Read the model definition and answer for the solid it produces. Units are mm, in the model's axes. Face numbers are marked on the shaded views. A direction names the side the tool comes from. Coordinates: 2 decimals unless noted, no trailing zeros. Loops run counter-clockwise (first coordinate to the right, second up) from the corner with the lowest first, then second, coordinate; pieces in that order, holes last. Notation, with made-up numbers: (51, -16) - (56, -16) arc R7 cw to (56, -10) - close; hole circle Ø11 at (76.5, -23). An arc over 180 degrees is marked (long way). Use one line per item in the form item = value.
from build123d import *

# Parameters (mm, degrees)
SKETCH1_W           = 30.86
SKETCH1_H           = 42.11
BOSS_EXTRUDE1_DEPTH = 10
SHELL2_T            = -2
SKETCH4_W           = 19.06
SKETCH4_H           = 2
CUT_EXTRUDE1_DEPTH  = 4
FILLET1_R           = 0.25
SKETCH5_R           = 1.5
CUT_EXTRUDE2_DEPTH  = 28.953495756
SKETCH6_R           = 1.5
CUT_EXTRUDE3_DEPTH  = 28.953495756


with BuildPart() as part:
    # Sketch1 → Boss-Extrude1 (new body)
    with BuildSketch(Plane(origin=(0, 0, 0), x_dir=(1, 0, 0), z_dir=(0, 1, 0))):
        Rectangle(SKETCH1_W, SKETCH1_H)
    extrude(amount=BOSS_EXTRUDE1_DEPTH)

    # Shell2
    shell2_openings = [part.faces().sort_by_distance(p)[0] for p in [
        (0, 10, 0),
    ]]
    offset(amount=SHELL2_T, openings=shell2_openings, kind=Kind.INTERSECTION)

    # Sketch4 → Cut-Extrude1 (cut)
    with BuildSketch(Plane(origin=(0, 10, 0), x_dir=(1, 0, 0), z_dir=(0, 1, 0))):
        with Locations((-3.9, -20.055)):
            Rectangle(SKETCH4_W, SKETCH4_H)
    extrude(amount=-CUT_EXTRUDE1_DEPTH, mode=Mode.SUBTRACT)

    # Fillet1
    fillet1_edges = [part.edges().sort_by_distance(p)[0] for p in [
        (0, 0, 21.055),
        (-15.43, 0, 0),
        (0, 0, -21.055),
        (15.43, 0, 0),
        (15.43, 5, 21.055),
        (-15.43, 5, 21.055),
        (-15.43, 5, -21.055),
        (15.43, 5, -21.055),
    ]]
    fillet(fillet1_edges, radius=FILLET1_R)

    # Sketch5 → Cut-Extrude2 (cut, through all)
    with BuildSketch(Plane.XZ):
        with Locations(Location((3.955545026, 15.646822422, 0), (0, 0, 270))):
            Circle(SKETCH5_R)
    extrude(amount=-CUT_EXTRUDE2_DEPTH, mode=Mode.SUBTRACT)

    # Sketch6 → Cut-Extrude3 (cut, through all)
    with BuildSketch(Plane.XZ):
        with Locations(Location((8.578599531, 12.725824803, 0), (0, 0, 270))):
            Circle(SKETCH6_R)
    extrude(amount=-CUT_EXTRUDE3_DEPTH, mode=Mode.SUBTRACT)


solid = part.part
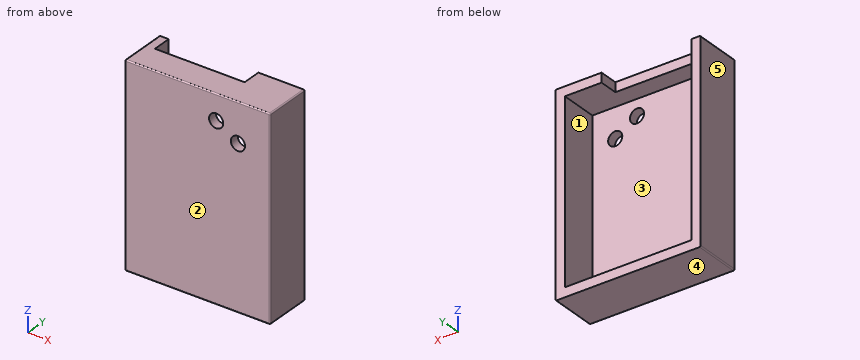
Item 1: Which of the six approach directions +Z, -Z, +X, -X, +Y, -Y give full straight-line access (tool end or side, diameter ignored) to the marked faces 1 and 2?
Results below:
face_1 = +Y
face_2 = +Z, -Z, +X, -X, -Y
Item 2: Each of these flat-tipped pins is pushed along its axis until it touches: P1, Ø5, axis at x = 8.58, z = 12.73, coming from the +Y side; P2, Ø1, axis at x = -7, z = 20, coming from the +Y side. Where does it stop, or does it pass through?
Results below:
P1 = 2
P2 = 6
Item 3: The part is cut by section B-B on y = 8.25. Give the vertices of the cut face in (x, z) (3 decimals).
Results below:
outline = (-15.43, -20.805) arc R0.25 ccw to (-15.18, -21.055) - (15.18, -21.055) arc R0.25 ccw to (15.43, -20.805) - (15.43, 20.805) arc R0.25 ccw to (15.18, 21.055) - (5.63, 21.055) - (5.63, 19.055) - (13.43, 19.055) - (13.43, -19.055) - (-13.43, -19.055) - (-13.43, 21.055) - (-15.18, 21.055) arc R0.25 ccw to (-15.43, 20.805) - close
Item 4: Find the intervals of material crossed by L1, parallel to X at y = 9.5, z = -18.5; L2, parallel to Z at x = 11, y = 7.25 (3 decimals); L3, parallel to Z at x = -1, y = 9.25 (3 decimals), in increasing order.
Results below:
L1 = -15.43 to -13.43, 13.43 to 15.43
L2 = -21.055 to -19.055, 19.055 to 21.055
L3 = -21.055 to -19.055
Item 5: For a pull along X with two mould halves and no side action, classify the marked faces 3, 4 and 5 as +X half, -X half, draft (parallel to the pull), parting line (faces both ways), or undercut.
Results below:
face_3 = undercut
face_4 = draft
face_5 = -X half
Item 6: The part is cut by section D-D on z = 7.5. Give the vertices of the cut face in (x, y), plus the area to 3 significant figures.
Results below:
outline = (-15.43, 0.25) arc R0.25 ccw to (-15.18, 0) - (15.18, 0) arc R0.25 ccw to (15.43, 0.25) - (15.43, 10) - (13.43, 10) - (13.43, 2) - (-13.43, 2) - (-13.43, 10) - (-15.43, 10) - close
area = 93.7 mm²
Item 7: The part is cut by section A-A on y = 3.75. Give the vertices of the cut face in (x, z) (3 decimals).
Results below:
outline = (-15.43, -20.805) arc R0.25 ccw to (-15.18, -21.055) - (15.18, -21.055) arc R0.25 ccw to (15.43, -20.805) - (15.43, 20.805) arc R0.25 ccw to (15.18, 21.055) - (-15.18, 21.055) arc R0.25 ccw to (-15.43, 20.805) - close; hole (-13.43, -19.055) - (13.43, -19.055) - (13.43, 19.055) - (-13.43, 19.055) - close
Item 8: The part is cut by section C-C on x = -7. Give the vertices of the cut face in (y, z) (3 decimals).
Results below:
outline = (0, -20.805) arc R0.25 ccw to (0.25, -21.055) - (10, -21.055) - (10, -19.055) - (2, -19.055) - (2, 19.055) - (6, 19.055) - (6, 21.055) - (0.25, 21.055) arc R0.25 ccw to (0, 20.805) - close
